Work out the finished part from the listing and answer in its coordinate system (mm). Face numbers are marked on the shaded views. Round coordinates to 2 decimals unless told otherwise and drop trailing zeros. Write each loop counter-clockwise with the first axis right and the second up, starting at its lowest first coordinate (ties: lowest second). Pieces come first, ordered by that corner, then holes.
1. Find section A-A (z = 8.25). Write down the section's boundary in (x, y).
2. Flat-ended cylindrical pins translate along their axes: pin 1 Ø2 at (x, y) = (-0.5, 6) entering from +Z; pin 2 Ø5 at (x, z) = (-2, 3) entering from -Y; pin 3 Ø1 at (x, z) = (3, 2.5) entering from -Y; pin 4 Ø1 at (x, z) = (1.5, 6.5) entering from +Y (3 decimals). Find the tip coordinate at first contact, or state that the pin passes through.
3. Straight lines are drawn through the part: probe 1 along X at (y, z) = (-0.75, 3.25); probe 2 along Y at (x, z) = (-0.25, 8.5); probe 3 along X at (y, z) = (1, 3). For each, find the intervals that lie inside material, in ascending order.
4. Determine the mould class of the marked faces 1, 2 and 3 for opening direction X: pulls with the +X half, pulls with the -X half, needs draft (parallel to the pull), parting line crosses it, or undercut.
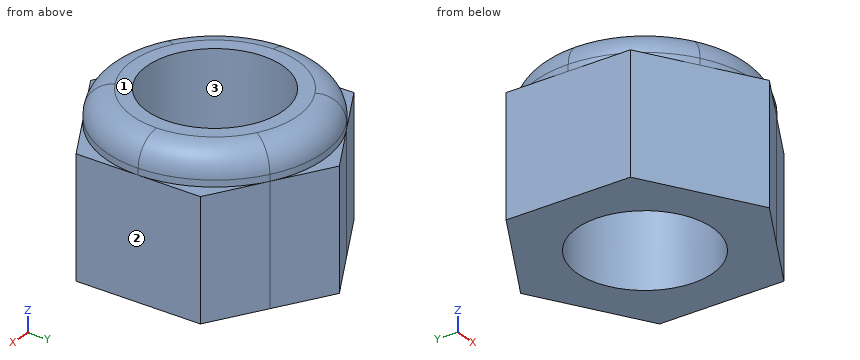
```python
from build123d import *

# Parameters (mm, degrees)
F0_R     = 3.96875
F1_DEPTH = 6.985
F2_DEPTH = 8.89
F3_R     = 1.524


with BuildPart() as f1:
    # F0 (on Top) → F1 (new body)
    with BuildSketch(Plane.XY):
        with BuildLine():
            Line((-6.35, -3.6661742094), (-3.174999936, -5.499261351))
            ThreePointArc((-3.174999936, -5.499261351), (-5.4992612955, -3.175000032), (-6.35, 0))
            Line((-6.35, 0), (-6.35, -3.6661742094))
        make_face()
        with BuildLine():
            ThreePointArc((-6.35, 0), (-5.4992613406, 3.174999954), (-3.175000092, 5.4992612609))
            Line((-3.175000092, 5.4992612609), (-6.35, 3.6661742094))
            Line((-6.35, 3.6661742094), (-6.35, 0))
        make_face()
        with BuildLine():
            ThreePointArc((-3.175000092, 5.4992612609), (-1.72e-08, 6.35), (3.1750000622, 5.4992612781))
            Line((3.1750000622, 5.4992612781), (0, 7.3323484187))
            Line((0, 7.3323484187), (-3.175000092, 5.4992612609))
        make_face()
        with BuildLine():
            ThreePointArc((3.1750000622, 5.4992612781), (5.499261332, 3.1749999689), (6.35, 0))
            Line((6.35, 0), (6.35, 3.6661742094))
            Line((6.35, 3.6661742094), (3.1750000622, 5.4992612781))
        make_face()
        with BuildLine():
            Line((6.35, -3.6661742094), (6.35, 0))
            ThreePointArc((6.35, 0), (5.4992613128, -3.1750000022), (3.1749999956, -5.4992613166))
            Line((3.1749999956, -5.4992613166), (6.35, -3.6661742094))
        make_face()
        with BuildLine():
            Line((0, -7.3323484187), (3.1749999956, -5.4992613166))
            ThreePointArc((3.1749999956, -5.4992613166), (3.44e-08, -6.35), (-3.174999936, -5.499261351))
            Line((-3.174999936, -5.499261351), (0, -7.3323484187))
        make_face()
        with BuildLine():
            ThreePointArc((3.1749999956, -5.4992613166), (5.4992613128, -3.1750000022), (6.35, 0))
            ThreePointArc((6.35, 0), (5.499261332, 3.1749999689), (3.1750000622, 5.4992612781))
            ThreePointArc((3.1750000622, 5.4992612781), (-1.72e-08, 6.35), (-3.175000092, 5.4992612609))
            ThreePointArc((-3.175000092, 5.4992612609), (-5.4992613406, 3.174999954), (-6.35, 0))
            ThreePointArc((-6.35, 0), (-5.4992612955, -3.175000032), (-3.174999936, -5.499261351))
            ThreePointArc((-3.174999936, -5.499261351), (3.44e-08, -6.35), (3.1749999956, -5.4992613166))
        make_face()
        Circle(F0_R, mode=Mode.SUBTRACT)
    extrude(amount=F1_DEPTH)

    # F0 (on Top) → F2 (join)
    with BuildSketch(Plane.XY):
        with BuildLine():
            ThreePointArc((3.1749999956, -5.4992613166), (5.4992613128, -3.1750000022), (6.35, 0))
            ThreePointArc((6.35, 0), (5.499261332, 3.1749999689), (3.1750000622, 5.4992612781))
            ThreePointArc((3.1750000622, 5.4992612781), (-1.72e-08, 6.35), (-3.175000092, 5.4992612609))
            ThreePointArc((-3.175000092, 5.4992612609), (-5.4992613406, 3.174999954), (-6.35, 0))
            ThreePointArc((-6.35, 0), (-5.4992612955, -3.175000032), (-3.174999936, -5.499261351))
            ThreePointArc((-3.174999936, -5.499261351), (3.44e-08, -6.35), (3.1749999956, -5.4992613166))
        make_face()
        Circle(F0_R, mode=Mode.SUBTRACT)
    extrude(amount=F2_DEPTH)

    # F3
    f3_edges = [f1.edges().sort_by_distance(p)[0] for p in [
        (3.175, -5.499261, 8.89),
    ]]
    fillet(f3_edges, radius=F3_R)


solid = f1.part
```
Worked answers:
1. outline: circle Ø12.13 at (0, 0); hole circle Ø7.94 at (0, 0)
2. pin 1: stops at z = 8.88
2. pin 2: stops at y = -7.33
2. pin 3: stops at y = -5.89
2. pin 4: stops at y = 6.755
3. probe 1: x = -6.35 to -3.9, 3.9 to 6.35
3. probe 2: y = -5.84 to -3.96, 3.96 to 5.84
3. probe 3: x = -6.35 to -3.84, 3.84 to 6.35
4. face 1: needs draft
4. face 2: pulls with the +X half
4. face 3: undercut
